Build history of the part. All positions in model axes, mm. A direction names the side the tool comes from. Round coordinates to 2 decimals unless told otherwise and drop trailing zeros. Loops run counter-clockwise (first coordinate to the right, second up) from the corner with the lowest first, then second, coordinate; pieces in that order, holes last. Notation, with made-up numbers: M 81,16 L 88,16 A19 cw 88,34 Z; hole C 63.25,-15 d6. An arc over 180 degrees is marked long. One line per item, written item: value.
```python
from build123d import *

# Parameters (mm, degrees)
SKETCH_1_R          = 12.9
EXTRUDE_1_DEPTH     = 31
SKETCH_2_R          = 8
CUT_EXTRUDE_1_DEPTH = 25
CHAMFER_1_SIZE      = 5
FILLET_1_R          = 1
SKETCH_3_W          = 3
SKETCH_3_H          = 3


with BuildPart() as part:
    # 草图1 → 凸台-拉伸1 (new body)
    with BuildSketch(Plane(origin=(0, 0, 0), x_dir=(1, 0, 0), z_dir=(0, 1, 0))):
        with Locations(Location((0, 0, 0), (0, 0, 270))):
            Circle(SKETCH_1_R)
    extrude(amount=EXTRUDE_1_DEPTH)

    # 草图2 → 切除-拉伸1 (cut)
    with BuildSketch(Plane(origin=(0, 31, 0), x_dir=(1, 0, 0), z_dir=(0, 1, 0))):
        with Locations(Location((0, 0, 0), (0, 0, 270))):
            Circle(SKETCH_2_R)
    extrude(amount=-CUT_EXTRUDE_1_DEPTH, mode=Mode.SUBTRACT)

    # 倒角1
    chamfer_1_edges = [part.edges().sort_by_distance(p)[0] for p in [
        (0, 0, -12.9),
    ]]
    chamfer(chamfer_1_edges, length=CHAMFER_1_SIZE)

    # 圆角1
    fillet_1_edges = [part.edges().sort_by_distance(p)[0] for p in [
        (0, 0, -7.9),
        (0, 5, -12.9),
    ]]
    fillet(fillet_1_edges, radius=FILLET_1_R)

    # 草图3 → 切除-旋转1 (revolve, cut)
    with BuildSketch(Plane.XY, mode=Mode.PRIVATE) as cut_revolve_1_sk:
        with Locations((11.4, 26.5)):
            Rectangle(SKETCH_3_W, SKETCH_3_H)
        with Locations((11.4, 20.5)):
            Rectangle(SKETCH_3_W, SKETCH_3_H)
        with Locations((11.4, 14.5)):
            Rectangle(SKETCH_3_W, SKETCH_3_H)
        with Locations((11.4, 8.5)):
            Rectangle(SKETCH_3_W, SKETCH_3_H)
    revolve(cut_revolve_1_sk.sketch.rotate(Axis((0, 0, 0), (0, 1, 0)), 90), axis=Axis((0, 0, 0), (0, 1, 0)), mode=Mode.SUBTRACT)


solid = part.part
```
Item 1: Pull direction X, two halves, no side cores. Call faces 3 (the face through (-7.81, 18.68, -1.73)), 4 (the face through (8, 25, 7)), 5 (the face through (0, 6, 0)), 6 (the face through (-11.445, 6.196, 5.953)): pulls with the +X half, pulls with the -X half, needs draft (parallel to the pull), parting line crosses it, or undercut.
Check values:
face 3: undercut
face 4: needs draft
face 5: undercut
face 6: parting line crosses it
Item 2: Drop flat-ended pins along their axis: P1, Ø1.5, axis at x = 1.5, y = 14.5, coming from the +Z side; P2, Ø3, axis at x = 3, y = 13, coming from the -Z side; P3, Ø1.5, axis at x = 0.5, z = -9.5, coming from the -Y side. Give the stop position or say it passes through.
Check values:
P1: stops at z = 9.87
P2: stops at z = -12.81
P3: stops at y = 0.86
Item 3: Which spindle directions (+Z, -Z, +X, -X, +Y, -Y) get a long thin tool onto all of the face, cutting with end or side? Do faces 1 (the face through (-12.593, 29.479, -2.796)), 2 (the face through (8, 16, 7)). Say none if no direction does.
Check values:
face 1: +Y, -Y
face 2: none
Item 4: Wall check: line 1 along Y through (x, z) = (8.5, 8); line 2 along Y through (x, z) = (8.5, -9); line 3 along Y through (x, z) = (1.5, 6.5). Give the ranges that are in metal, low to high.
Check values:
line 1: y = 3.77 to 7, 10 to 13, 16 to 19, 22 to 25, 28 to 31
line 2: y = 4.48 to 7, 10 to 13, 16 to 19, 22 to 25, 28 to 31
line 3: y = 0 to 6
Item 5: Slice it at A-A, the plane y = 18. Give the cut face in (x, z).
Check values:
outline: C 0,0 d25.8; hole C 0,0 d16
